from build123d import *

# Parameters (mm, degrees)
SKETCH1_R           = 38.1
BOSS_EXTRUDE1_DEPTH = 3
SKETCH3_R           = 1.778
CUT_EXTRUDE1_DEPTH  = 54.96498865
CIRPATTERN1_COUNT   = 4
CUT_EXTRUDE2_DEPTH  = 54.96498865


with BuildPart() as part:
    # Sketch1 → Boss-Extrude1 (new body)
    with BuildSketch(Plane(origin=(0, 0, 0), x_dir=(1, 0, 0), z_dir=(0, 1, 0))):
        with Locations(Location((0, 0, 0), (0, 0, 270))):
            Circle(SKETCH1_R)
    extrude(amount=BOSS_EXTRUDE1_DEPTH)

    # Sketch3 → Cut-Extrude1 (cut, through all)
    with BuildSketch(Plane(origin=(0, 3, 0), x_dir=(1, 0, 0), z_dir=(0, 1, 0))):
        with Locations(Location((33.02, 0, 0), (0, 0, 270))):
            Circle(SKETCH3_R)
    cut_extrude1 = extrude(amount=-CUT_EXTRUDE1_DEPTH, mode=Mode.SUBTRACT)

    # CirPattern1: Cut-Extrude1 ×4 about axis
    cirpattern1_axis = Axis((0, 0, 0), (0, 1, 0))
    for i in range(1, CIRPATTERN1_COUNT):
        add(cut_extrude1.rotate(cirpattern1_axis, i * 360 / CIRPATTERN1_COUNT), mode=Mode.SUBTRACT)

    # Sketch4 → Cut-Extrude2 (cut, through all)
    with BuildSketch(Plane(origin=(0, 3, 0), x_dir=(1, 0, 0), z_dir=(0, 1, 0))):
        with BuildLine():
            Line((-2.598076211, 1.5), (2.598076211, 1.5))
            ThreePointArc((2.598076211, 1.5), (0, -3), (-2.598076211, 1.5))
        make_face()
    extrude(amount=-CUT_EXTRUDE2_DEPTH, mode=Mode.SUBTRACT)


solid = part.part
Input: part model. Units: mm. Frame: model coordinates. A direction names the side the tool comes from. Coordinates: 2 decimals unless noted, no trailing zeros. Loops run counter-clockwise (first coordinate to the right, second up) from the corner with the lowest first, then second, coordinate; pieces in that order, holes last.
Q1. Cut plane C-C (x = 0). Output: boundary loops of the cut face in (y, z), then the cut area to 3 significant figures.
Q2. Draft query along X for faces 1 (the face through (-23.183, 1.479, -30.235)), 2 (the face through (1, 3, 8)), 3 (the face through (-34.783, 1.521, 0.231)), 4 (the face through (-0.231, 1.521, -34.783)). Return one class per face: +X half, -X half, draft (parallel to the pull), parting line (faces both ways), or undercut.
Q3. Cut plane B-B (y = 2.5). Output: boundary loops of the cut face in (x, z), then the cut area to 3 significant figures.
Q4. Cut plane D-D (x = -33.02). Output: boundary loops of the cut face in (y, z).
Q5. Cut plane A-A (z = 0). Output: boundary loops of the cut face in (x, y), then the cut area to 3 significant figures.
Q6. Material intervals for line 1 (X direction, y = 2.15, z = 0); line 2 (X direction, y = 0.2, z = -1); line 3 (X direction, y = 1.6, z = -34.5), sorted ascending.
Q7. Set-up query: faces 5 (the face through (1, 0, 8)), 6 (the face through (0, 2, -1.5)). Return all of +Z, -Z, +X, -X, +Y, -Y with unobstructed straight access to the full face (end or side cutting, diameter ignored); none if empty.
Q8. Contact query for flat-ended pins moving along their axis: pin 1 (4 mm diameter, centred on x = 0, z = 33.02, fed in from -Y); pin 2 (1.5 mm diameter, centred on x = -13, y = 2.5, fed in from -Z); pin 3 (1.5 mm diameter, centred on x = -24, y = 2.5, fed in from -Z). Output: stop coordinate, or through.
Working result:
1. outline: (0, -38.1) - (3, -38.1) - (3, -34.8) - (0, -34.8) - close; (0, -31.24) - (3, -31.24) - (3, -1.5) - (0, -1.5) - close; (0, 3) - (3, 3) - (3, 31.24) - (0, 31.24) - close; (0, 34.8) - (3, 34.8) - (3, 38.1) - (0, 38.1) - close
1. area: 194 mm2
2. face 1: parting line
2. face 2: draft
2. face 3: undercut
2. face 4: undercut
3. outline: circle Ø76.2 at (0, 0); hole circle Ø3.56 at (-33.02, 0); hole (-2.6, -1.5) - (2.6, -1.5) arc R3 ccw (long way) to start; hole circle Ø3.56 at (0, -33.02); hole circle Ø3.56 at (0, 33.02); hole circle Ø3.56 at (33.02, 0)
3. area: 4,500 mm2
4. outline: (0, -19.01) - (3, -19.01) - (3, -1.78) - (0, -1.78) - close; (0, 1.78) - (3, 1.78) - (3, 19.01) - (0, 19.01) - close
5. outline: (-38.1, 0) - (-34.8, 0) - (-34.8, 3) - (-38.1, 3) - close; (-31.24, 0) - (-3, 0) - (-3, 3) - (-31.24, 3) - close; (3, 0) - (31.24, 0) - (31.24, 3) - (3, 3) - close; (34.8, 0) - (38.1, 0) - (38.1, 3) - (34.8, 3) - close
5. area: 189 mm2
6. line 1: x = -38.1 to -34.8, -31.24 to -3, 3 to 31.24, 34.8 to 38.1
6. line 2: x = -38.09 to -34.49, -31.55 to -2.83, 2.83 to 31.55, 34.49 to 38.09
6. line 3: x = -16.17 to -0.99, 0.99 to 16.17
7. face 5: +Z, -Z, +X, -X, -Y
7. face 6: +Y, -Y
8. pin 1: stops at y = 0
8. pin 2: stops at z = -36.08
8. pin 3: stops at z = -30.18
